Drawing for the job (mm, zero at the part's lowest x, y, z). A direction names the side the tool comes from. Round coordinates to 2 decimals unless told otherwise and drop trailing zeros. Order: outer loops, then holes, each group sorted by start corner. A loop starts at its lowest first (then second) coordinate and runs counter-clockwise, first axis right, second up. Notation, with made-up numbers: (6, -18.75) -> (14, -18.75) arc R16 cw to (14, -4.75) -> close; hole circle Ø8 at (23, 88.25). An arc over 180 degrees is marked (long way). Use CSV: the item, a comma, the result in double quotes.
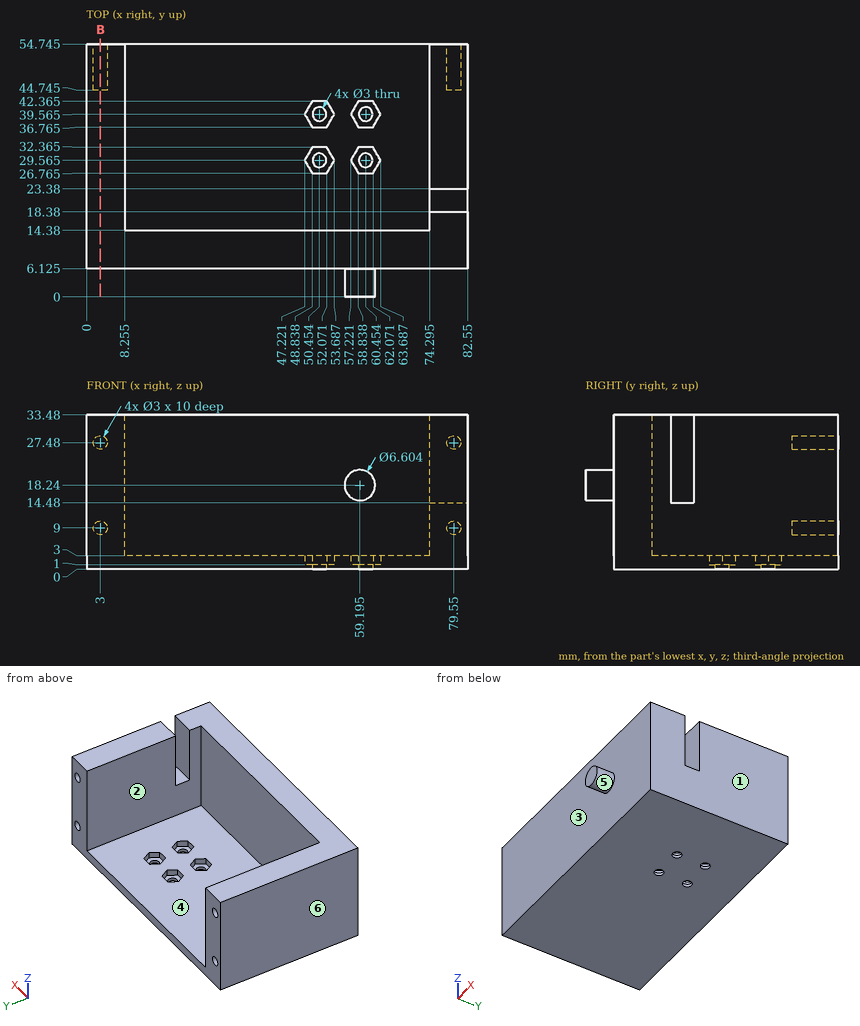
Q1. Pin check, flat tips, straight feed: pin 1 (6 mm diameter, centred on x = 60, y = 20, fed in from +Z); pin 2 (1.5 mm diameter, centred on x = 80, z = 27, fed in from +Y) (3 decimals); pin 3 (3.5 mm diameter, centred on x = 2.5, z = 9.5, fed in from +Y) (3 decimals); pin 4 (3.5 mm diameter, centred on x = 50.45, y = 29.56, fed in from +Z). Stop position of each tip, or through.
From the geometry:
pin 1,"stops at z = 3"
pin 2,"stops at y = 44.745"
pin 3,"stops at y = 54.745"
pin 4,"stops at z = 1"
Q2. Cut at B-B (x = 3). Give the cut face in (y, z) (1 decimal), plus the area to 3 significant figures.
From the geometry:
outline,"(6.1, 0) -> (54.7, 0) -> (54.7, 7.5) -> (44.7, 7.5) -> (44.7, 10.5) -> (54.7, 10.5) -> (54.7, 26) -> (44.7, 26) -> (44.7, 29) -> (54.7, 29) -> (54.7, 33.5) -> (6.1, 33.5) -> close"
area,"1,570 mm²"
Q3. Mould opens along X. For the marked faces 1, 2 and 3 say: +X half, -X half, draft (parallel to the pull), parting line (faces both ways), or undercut.
From the geometry:
face 1,"+X half"
face 2,"undercut"
face 3,"draft"
Q4. Probe line 1 along Z through (x, y) = (3, 50.25); line 2 along Z through (x, y) = (79, 49) (1 decimal); line 3 along Y through (x, z) = (26, 18) (1 decimal). List the from-to ranges inside material, lowest first.
From the geometry:
line 1,"z = 0 to 7.5, 10.5 to 25.98, 28.98 to 33.48"
line 2,"z = 0 to 7.6, 10.4 to 26.1, 28.9 to 33.5"
line 3,"y = 6.1 to 14.4"
Q5. Which spindle directions (+Z, -Z, +X, -X, +Y, -Y) get a long thin tool onto all of the face, cutting with end or side? Do the marked faces 4, 5 and 6. Say none if no direction does.
From the geometry:
face 4,"+Z, +Y"
face 5,"-Y"
face 6,"+Z, -Z, -X, +Y, -Y"
